Read the model definition and answer for the solid it produces. Units are mm, in the model's axes. A direction names the side the tool comes from. Coordinates: 2 decimals unless noted, no trailing zeros. Order: outer loops, then holes, each group sorted by start corner. A loop starts at its lowest first (then second) coordinate and runs counter-clockwise, first axis right, second up.
```python
from build123d import *

# Parameters (mm, degrees)
F0_R     = 3.175
F0_R_2   = 5.1
F1_DEPTH = 6


with BuildPart() as f1:
    # F0 (on Front) → F1 (new body)
    with BuildSketch(Plane.XZ):
        with BuildLine():
            Line((368.3, 36.3), (368.3, 53.8))
            ThreePointArc((368.3, 53.8), (366.835534, 57.335534), (363.3, 58.8))
            Line((363.3, 58.8), (289.998539, 58.8))
            ThreePointArc((289.998539, 58.8), (279.391937, 54.406602), (274.998539, 43.8))
            Line((274.998539, 43.8), (274.998539, 15))
            ThreePointArc((274.998539, 15), (270.605141, 4.393398), (259.998539, 0))
            Line((259.998539, 0), (0, 0))
            Line((0, 0), (-259.998539, 0))
            ThreePointArc((-259.998539, 0), (-270.605141, 4.393398), (-274.998539, 15))
            Line((-274.998539, 15), (-274.998539, 43.8))
            ThreePointArc((-274.998539, 43.8), (-279.391937, 54.406602), (-289.998539, 58.8))
            Line((-289.998539, 58.8), (-363.3, 58.8))
            ThreePointArc((-363.3, 58.8), (-366.835534, 57.335534), (-368.3, 53.8))
            Line((-368.3, 53.8), (-368.3, 36.3))
            ThreePointArc((-368.3, 36.3), (-366.532233, 35.567767), (-365.8, 33.8))
            ThreePointArc((-365.8, 33.8), (-368.3, 31.3), (-370.8, 33.8))
            Line((-370.8, 33.8), (-388.3, 33.8))
            ThreePointArc((-388.3, 33.8), (-391.835534, 32.335534), (-393.3, 28.8))
            Line((-393.3, 28.8), (-393.3, -90))
            ThreePointArc((-393.3, -90), (-388.906602, -100.606602), (-378.3, -105))
            Line((-378.3, -105), (0, -105))
            Line((0, -105), (378.3, -105))
            ThreePointArc((378.3, -105), (388.906602, -100.606602), (393.3, -90))
            Line((393.3, -90), (393.3, 28.8))
            ThreePointArc((393.3, 28.8), (391.835534, 32.335534), (388.3, 33.8))
            Line((388.3, 33.8), (370.8, 33.8))
            ThreePointArc((370.8, 33.8), (366.532233, 32.032233), (368.3, 36.3))
        make_face()
        with Locations((-254.7125, -68)):
            Circle(F0_R, mode=Mode.SUBTRACT)
        with Locations((-229.7125, -68)):
            Circle(F0_R, mode=Mode.SUBTRACT)
        with Locations((-204.7125, -68)):
            Circle(F0_R, mode=Mode.SUBTRACT)
        with Locations((-254.7125, -43)):
            Circle(F0_R, mode=Mode.SUBTRACT)
        with Locations((-185.6125, -26.9)):
            Circle(F0_R_2, mode=Mode.SUBTRACT)
        with BuildLine():
            ThreePointArc((-155.164491, -24.375544), (-149.556494, -20.75), (-143.948498, -24.375544))
            Line((-143.948498, -24.375544), (-139.556503, -24.375544))
            ThreePointArc((-139.556503, -24.375544), (-137.788736, -25.107777), (-137.056503, -26.875544))
            ThreePointArc((-137.056503, -26.875544), (-137.788736, -28.643311), (-139.556503, -29.375544))
            Line((-139.556503, -29.375544), (-143.926736, -29.375544))
            ThreePointArc((-143.926736, -29.375544), (-149.556494, -33.05), (-155.186253, -29.375544))
            Line((-155.186253, -29.375544), (-159.556503, -29.375544))
            ThreePointArc((-159.556503, -29.375544), (-162.056494, -26.87554), (-159.556494, -24.375544))
            Line((-159.556494, -24.375544), (-155.164491, -24.375544))
        make_face(mode=Mode.SUBTRACT)
        with Locations((204.7125, -68)):
            Circle(F0_R, mode=Mode.SUBTRACT)
        with Locations((229.7125, -68)):
            Circle(F0_R, mode=Mode.SUBTRACT)
        with Locations((254.7125, -68)):
            Circle(F0_R, mode=Mode.SUBTRACT)
        with BuildLine():
            ThreePointArc((143.948498, -24.375544), (149.556494, -20.75), (155.164491, -24.375544))
            Line((155.164491, -24.375544), (159.556494, -24.375544))
            ThreePointArc((159.556494, -24.375544), (161.324261, -25.107777), (162.056494, -26.875544))
            ThreePointArc((162.056494, -26.875544), (161.324264, -28.643308), (159.556503, -29.375544))
            Line((159.556503, -29.375544), (155.186253, -29.375544))
            ThreePointArc((155.186253, -29.375544), (149.556494, -33.05), (143.926736, -29.375544))
            Line((143.926736, -29.375544), (139.556503, -29.375544))
            ThreePointArc((139.556503, -29.375544), (137.056503, -26.875544), (139.556503, -24.375544))
            Line((139.556503, -24.375544), (143.948498, -24.375544))
        make_face(mode=Mode.SUBTRACT)
        with Locations((185.6125, -26.9)):
            Circle(F0_R_2, mode=Mode.SUBTRACT)
        with Locations((254.7125, -43)):
            Circle(F0_R, mode=Mode.SUBTRACT)
        with Locations((-254.7125, -18)):
            Circle(F0_R, mode=Mode.SUBTRACT)
        with Locations((-380.8, 13.8)):
            Circle(F0_R, mode=Mode.SUBTRACT)
        with Locations((-348.3, 13.8)):
            Circle(F0_R, mode=Mode.SUBTRACT)
        with Locations((-348.3, 46.3)):
            Circle(F0_R, mode=Mode.SUBTRACT)
        with Locations((254.7125, -18)):
            Circle(F0_R, mode=Mode.SUBTRACT)
        with Locations((348.3, 13.8)):
            Circle(F0_R, mode=Mode.SUBTRACT)
        with Locations((380.8, 13.8)):
            Circle(F0_R, mode=Mode.SUBTRACT)
        with Locations((348.3, 46.3)):
            Circle(F0_R, mode=Mode.SUBTRACT)
    extrude(amount=F1_DEPTH)


solid = f1.part
```
1) A cutting plane is placed at B-B, the plane x = 83.5. Determine the outline of the cut face in (y, z).
A:
outline: (-6, -105) - (0, -105) - (0, 0) - (-6, 0) - close
2) Straight lines are drawn through the part: line 1 (Z direction, x = -254, y = -1.85); line 2 (Z direction, x = 348.3, y = -3) (3 decimals); line 3 (Z direction, x = 219, y = -5.3). For each, find the intervals that lie inside material, in ascending order.
A:
line 1: z = -105 to -71.09, -64.91 to -46.09, -39.91 to -21.09, -14.91 to 0
line 2: z = -105 to 10.625, 16.975 to 43.125, 49.475 to 58.8
line 3: z = -105 to 0
3) A cutting plane is placed at A-A, the plane y = -4.3. State how many separate pieces and enclosed holes the cut face has, and give its area (3 significant figures).
A:
separate pieces: 1
enclosed holes: 20
area: 94,100 mm2
4) Which of the six approach directions +Z, -Z, +X, -X, +Y, -Y give full straight-line access (tool end or side, diameter ignored) to faces 1 (the flat face through (-6, 0, -40)), 2 (the cylindrical face through (279.509, -2.958, 54.523))?
A:
face 1: +Z, -Z, +X, -X, +Y
face 2: +Z, +Y, -Y
5) Flat-ended cylindrical pins translate along their axes: pin 1 Ø1 at (x, z) = (-201, -13.5) entering from +Y; pin 2 Ø5.5 at (x, z) = (254.71, -18) entering from -Y; pin 3 Ø2 at (x, y) = (-158, -3.5) entering from +Z; pin 4 Ø3 at (x, y) = (382.5, -4.5) entering from +Z. Find the tip coordinate at first contact, or state that the pin passes through.
A:
pin 1: stops at y = 0
pin 2: passes through
pin 3: stops at z = 0
pin 4: stops at z = 33.8
6) Determine the mould class of faces 3 (the flat face through (-6, -6, -40)), 4 (the cylindrical face through (-279, -3, 54)), 5 (the cylindrical face through (388.79, -2.96, -100.72)), 6 (the cylindrical face through (-270.49, -2.96, 4.28)) for opening direction X: pulls with the +X half, pulls with the -X half, needs draft (parallel to the pull), parting line crosses it, or undercut.
A:
face 3: needs draft
face 4: undercut
face 5: pulls with the +X half
face 6: undercut
